Work out the finished part from the listing and answer in its coordinate system (mm). A direction names the side the tool comes from. Give positions to 0.01 mm unless a question says otherwise; leave off trailing zeros. Loops run counter-clockwise (first coordinate to the right, second up) from the corner with the lowest first, then second, coordinate; pieces in that order, holes last. Notation, with made-up numbers: (26, 66) - (80, 66) arc R23 ccw to (80, 87) - close; hole circle Ø9 at (46.5, -17). An arc over 180 degrees is marked (long way). One line per item, written item: value.
from build123d import *

# Parameters (mm, degrees)
CROQUIS1_R              = 10.668000000000001
SALIENTE_EXTRUIR1_DEPTH = 5
CORTAR_EXTRUIR1_REACH   = 55.921
CROQUIS2_R              = 2.249999999999999
SALIENTE_EXTRUIR2_DEPTH = 2.5
CORTAR_EXTRUIR5_DEPTH   = 55.61204651906025
SALIENTE_EXTRUIR3_DEPTH = 10
CORTAR_EXTRUIR6_REACH   = 65.994
CROQUIS9_R              = 2.250000000000002
CORTAR_EXTRUIR7_DEPTH   = 60.57595316665593
SALIENTE_EXTRUIR4_DEPTH = 10
CROQUIS12_R             = 2.249999999999999
CORTAR_EXTRUIR8_DEPTH   = 10


with BuildPart() as part:
    # Croquis1 → Saliente-Extruir1 (new, symmetric)
    with BuildSketch(Plane(origin=(0, 0, 0), x_dir=(1, 0, 0), z_dir=(0, 1, 0))):
        with BuildLine():
            Line((30, 1.163e-14), (-30, -6.74e-15))
            Line((-30, -6.74e-15), (-29.999999999999993, -10.000000000000007))
            Line((-29.999999999999993, -10.000000000000007), (-4.999999999999997, -9.999999999999998))
            Line((-4.999999999999997, -9.999999999999998), (-4.999999999999997, -16.362711963150442))
            ThreePointArc((-4.999999999999997, -16.362711963150442), (1.01e-15, -44.525000000000006), (5.000000000000002, -16.362711963150442))
            Line((5.000000000000002, -16.362711963150442), (5.000000000000001, -9.999999999999993))
            Line((5.000000000000001, -9.999999999999993), (30, -9.999999999999988))
            Line((30, -9.999999999999988), (30, 1.163e-14))
        make_face()
        with Locations(Location((3.67e-15, -30, 0), (0, 0, 270))):
            Circle(CROQUIS1_R, mode=Mode.SUBTRACT)
    extrude(amount=SALIENTE_EXTRUIR1_DEPTH, both=True)

    # Croquis2 → Cortar-Extruir1 (cut, up to next)
    with BuildSketch(Plane(origin=(0, 0, 0), x_dir=(-1, 0, 3.1e-16), z_dir=(-3.1e-16, 0, -1)), mode=Mode.PRIVATE) as cortar_extruir1_sk1:
        with Locations((24.999999999999996, 0)):
            Circle(CROQUIS2_R)
    cortar_extruir1_tool1 = extrude(cortar_extruir1_sk1.sketch, amount=-CORTAR_EXTRUIR1_REACH, mode=Mode.PRIVATE) & part.part
    # Croquis2 → Cortar-Extruir1 (cut, up to next)
    with BuildSketch(Plane(origin=(0, 0, 0), x_dir=(-1, 0, 3.1e-16), z_dir=(-3.1e-16, 0, -1)), mode=Mode.PRIVATE) as cortar_extruir1_sk2:
        with Locations((-24.999999999999996, 0)):
            Circle(CROQUIS2_R)
    cortar_extruir1_tool2 = extrude(cortar_extruir1_sk2.sketch, amount=-CORTAR_EXTRUIR1_REACH, mode=Mode.PRIVATE) & part.part
    add(cortar_extruir1_tool1.solids().sort_by_distance((-25, 0, 0))[0], mode=Mode.SUBTRACT)
    add(cortar_extruir1_tool2.solids().sort_by_distance((25, 0, 0))[0], mode=Mode.SUBTRACT)

    # Croquis3 → Saliente-Extruir2 (add, symmetric)
    with BuildSketch(Plane(origin=(0, 0, 0), x_dir=(1, 0, 0), z_dir=(0, 1, 0))):
        with BuildLine():
            ThreePointArc((-4.999999999999991, -16.362711963150442), (-12.83879356101969, -23.207282951754927), (-14.087370599725464, -33.53858934972546))
            Line((-14.087370599725464, -33.53858934972546), (-19.999999999999996, -10.000000000000007))
            Line((-19.999999999999996, -10.000000000000007), (-4.999999999999997, -9.999999999999998))
            Line((-4.999999999999997, -9.999999999999998), (-4.999999999999991, -16.362711963150442))
        make_face()
        with BuildLine():
            Line((4.999999999999997, -9.999999999999998), (4.999999999999991, -16.362711963150442))
            ThreePointArc((4.999999999999991, -16.362711963150442), (12.838793561019703, -23.20728295175493), (14.087370599725464, -33.53858934972546))
            Line((14.087370599725464, -33.53858934972546), (19.999999999999996, -10.000000000000007))
            Line((19.999999999999996, -10.000000000000007), (4.999999999999997, -9.999999999999998))
        make_face()
    extrude(amount=SALIENTE_EXTRUIR2_DEPTH, both=True)

    # Croquis7 → Cortar-Extruir5 (cut, through all)
    with BuildSketch(Plane(origin=(0, 5, 0), x_dir=(1, 0, 0), z_dir=(0, 1, 0))):
        Polygon((1.0000000000000004, -46.5965), (-0.9999999999999998, -46.5965), (-0.9999999999999996, -38.5965), (1.0000000000000004, -38.5965), align=None)
    extrude(amount=-CORTAR_EXTRUIR5_DEPTH, mode=Mode.SUBTRACT)

    # Croquis8 → Saliente-Extruir3 (add)
    with BuildSketch(Plane(origin=(0, 5, 0), x_dir=(1, 0, 0), z_dir=(0, 1, 0))):
        with BuildLine():
            Line((-0.9999999999999998, -44.49053570438305), (-0.9999999999999989, -50.49053570438305))
            Line((-0.9999999999999989, -50.49053570438305), (-9, -50.490535704383056))
            Line((-9, -50.490535704383056), (-8.999999999999998, -41.400685286420284))
            ThreePointArc((-8.999999999999998, -41.400685286420284), (-5.233239331556143, -43.5494956031084), (-0.9999999999999998, -44.49053570438305))
        make_face()
        with BuildLine():
            Line((9, -50.490535704383056), (8.999999999999998, -41.400685286420284))
            ThreePointArc((8.999999999999998, -41.400685286420284), (5.23323933155614, -43.5494956031084), (0.9999999999999996, -44.49053570438305))
            Line((0.9999999999999996, -44.49053570438305), (0.9999999999999989, -50.49053570438305))
            Line((0.9999999999999989, -50.49053570438305), (9, -50.490535704383056))
        make_face()
    extrude(amount=-SALIENTE_EXTRUIR3_DEPTH)

    # Cortar-Extruir6: up to this face of the body (flat: up to its plane)
    cortar_extruir6_end = Plane(part.part.faces().sort_by_distance((-9, 0, 45.945610495))[0])
    # Croquis9 → Cortar-Extruir6 (cut, up to the picked face)
    with BuildSketch(Plane(origin=(8.99999999999999, 0, -1.72e-15), x_dir=(0, 0, -1), z_dir=(1, 0, 0)), mode=Mode.PRIVATE) as cortar_extruir6_sk1:
        with Locations((-45.945610495401674, 0)):
            Circle(CROQUIS9_R)
    cortar_extruir6_tool1 = split(extrude(cortar_extruir6_sk1.sketch, amount=-CORTAR_EXTRUIR6_REACH, mode=Mode.PRIVATE), bisect_by=cortar_extruir6_end, keep=Keep.BOTH, mode=Mode.PRIVATE)
    add(cortar_extruir6_tool1.solids().sort_by(Axis((9, 0, 45.94561), (-1, 0, 0)))[0], mode=Mode.SUBTRACT)

    # Croquis10 → Cortar-Extruir7 (cut, through all)
    with BuildSketch(Plane(origin=(0, 5, 0), x_dir=(1, 0, 0), z_dir=(0, 1, 0))):
        with BuildLine():
            ThreePointArc((-4.999999999999991, -16.362711963150442), (4.56e-15, -15.475), (5, -16.362711963150446))
            Line((5, -16.362711963150446), (5.000000000000001, -9.999999999999993))
            Line((5.000000000000001, -9.999999999999993), (30, -9.999999999999988))
            Line((30, -9.999999999999988), (30, 1.163e-14))
            Line((30, 1.163e-14), (-30, -6.74e-15))
            Line((-30, -6.74e-15), (-29.999999999999993, -10.000000000000007))
            Line((-29.999999999999993, -10.000000000000007), (-4.999999999999997, -9.999999999999998))
            Line((-4.999999999999997, -9.999999999999998), (-4.999999999999991, -16.362711963150442))
        make_face()
        with BuildLine():
            ThreePointArc((-14.087370599725464, -33.53858934972547), (-12.838793561019695, -23.207282951754934), (-4.999999999999991, -16.362711963150442))
            Line((-4.999999999999991, -16.362711963150442), (-4.999999999999997, -9.999999999999998))
            Line((-4.999999999999997, -9.999999999999998), (-20, -10.000000000000004))
            Line((-20, -10.000000000000004), (-14.087370599725462, -33.53858934972547))
        make_face()
        with BuildLine():
            Line((20.000000000000004, -9.99999999999999), (5, -9.999999999999993))
            Line((5.000000000000001, -9.999999999999993), (5.000000000000002, -16.362711963150442))
            ThreePointArc((5, -16.36271196315044), (12.838793561019697, -23.207282951754934), (14.08737059972547, -33.53858934972546))
            Line((14.087370599725467, -33.53858934972546), (20.000000000000004, -9.99999999999999))
        make_face()
    extrude(amount=-CORTAR_EXTRUIR7_DEPTH, mode=Mode.SUBTRACT)

    # Croquis11 → Saliente-Extruir4 (add)
    with BuildSketch(Plane(origin=(0, 5, 0), x_dir=(1, 0, 0), z_dir=(0, 1, 0))):
        with BuildLine():
            Line((29.525000000000002, -34.99999999999999), (29.525, -25))
            Line((29.525, -25), (13.637288036849554, -25))
            ThreePointArc((13.637288036849554, -25), (14.525, -30), (13.637288036849556, -35))
            Line((13.637288036849556, -35), (29.525000000000002, -34.99999999999999))
        make_face()
        with BuildLine():
            Line((-29.525000000000002, -34.99999999999999), (-13.637288036849556, -35))
            ThreePointArc((-13.637288036849556, -35), (-14.525, -30.000000000000004), (-13.637288036849554, -25))
            Line((-13.637288036849554, -25), (-29.525, -25))
            Line((-29.525, -25), (-29.525000000000002, -34.99999999999999))
        make_face()
    extrude(amount=-SALIENTE_EXTRUIR4_DEPTH)

    # Croquis12 → Cortar-Extruir8 (cut)
    with BuildSketch(Plane(origin=(29.524999999999988, 0, -1.024e-14), x_dir=(-3.5e-16, 0, -1), z_dir=(1, 0, -3.5e-16))):
        with Locations((-30.000000000000007, -8.7e-16)):
            Circle(CROQUIS12_R)
    cortar_extruir8 = extrude(amount=-CORTAR_EXTRUIR8_DEPTH, mode=Mode.SUBTRACT)

    # Simetría1: Cortar-Extruir8 across plane
    add(cortar_extruir8.mirror(Plane(origin=(0, 0, 0), x_dir=(0, 0, 1), z_dir=(1, 0, 0))), mode=Mode.SUBTRACT)


solid = part.part
1. Section B-B (y = 0) is taken. Count the separate pieces of the cut face and the enclosed holes in it, and give its area (3 significant figures).
Output:
separate pieces: 3
enclosed holes: 0
area: 555 mm²
2. Find the intervals of material crossed by line 1 along X through (y, z) = (1.25, 30) (3 decimals); line 2 along Y through (x, z) = (24.75, 30); line 3 along X through (y, z) = (-1.5, 43), in increasing order.
Output:
line 1: x = -19.525 to -10.668, 10.668 to 19.525
line 2: y = -5 to -2.25, 2.25 to 5
line 3: x = -9 to -1, 1 to 9
3. Section C-C (x = 22) is taken. Write down the section's boundary in (y, z).
Output:
outline: (-5, 25) - (5, 25) - (5, 35) - (-5, 35) - close; hole circle Ø4.5 at (0, 30)
4. For faces 5 (the flat face through (-9, 2.3, 47)), 6 (the flat face through (22, 0, 25)), 7 (the flat face through (21, 0, 35)), 8 (the flat face through (19.525, 0, 30)), 9 (the flat face through (-21, 0, 25)), determine the directions among +Z, -Z, +X, -X, +Y, -Y from which every point of the face is accessible in a straight line to the end or side of a thin tool.
Output:
face 5: +Z, -X, +Y, -Y
face 6: -Z, +X, +Y, -Y
face 7: +Z, +X, +Y, -Y
face 8: +X
face 9: -Z, -X, +Y, -Y
5. Section D-D (y = -3) is taken. Write down the section's boundary in (x, z) (3 decimals).
Output:
outline: (-29.525, 25) - (-13.637, 25) arc R14.525 ccw to (13.637, 25) - (29.525, 25) - (29.525, 35) - (13.637, 35) arc R14.525 ccw to (9, 41.401) - (9, 50.491) - (1, 50.491) - (1, 40.621) arc R10.668 cw (long way) to (-1, 40.621) - (-1, 50.491) - (-9, 50.491) - (-9, 41.401) arc R14.525 ccw to (-13.637, 35) - (-29.525, 35) - close
6. Flat-ended cylindrical pins translate along their axes: pin 1 Ø2.5 at (y, z) = (2.5, 43.5) entering from -X; pin 2 Ø4 at (y, z) = (-3.5, 43) entering from -X; pin 3 Ø4 at (y, z) = (-1.5, 43) entering from +X. Find the tip coordinate at first contact, or state that the pin passes through.
Output:
pin 1: stops at x = -9
pin 2: stops at x = -9.49
pin 3: stops at x = 9.49
7. Section A-A (z = 30) is taken. Write down the section's boundary in (x, y) (3 decimals).
Output:
outline: (-29.525, -5) - (-10.668, -5) - (-10.668, 5) - (-29.525, 5) - (-29.525, 2.25) - (-19.525, 2.25) - (-19.525, -2.25) - (-29.525, -2.25) - close; (10.668, -5) - (29.525, -5) - (29.525, -2.25) - (19.525, -2.25) - (19.525, 2.25) - (29.525, 2.25) - (29.525, 5) - (10.668, 5) - close
8. The mould has two halves that part along X. Classify faces 1 (the flat face through (29.525, 2.3, 31.2)), 2 (the flat face through (1, 0, 43)), 3 (the cylindrical face through (5.06, 0.68, 43.8)), 4 (the flat face through (-1, 0, 43)): released by +X, released by -X, zero draft, split by the parting line, or undercut.
Output:
face 1: released by +X
face 2: undercut
face 3: zero draft
face 4: undercut
